Geometry check sheet. Reference: drawing and pictorial views, mm from the part's lowest x, y, z. Coordinates: 2 decimals unless noted, no trailing zeros. Order: outer loops, then holes, each group sorted by start corner. A loop starts at its lowest first (then second) coordinate and runs counter-clockwise, first axis right, second up. Notation, with made-up numbers: (85, 42.25) -> (99, 42.25) arc R21 ccw to (99, 52.25) -> close; hole circle Ø8 at (34, 34.5). An arc over 180 degrees is marked (long way). Use CSV: the item, a comma, the result in double quotes. Start each with the question number.
1) Sectioned sample at A-A on z = 3.75. Record the boundary of the cut face in (x, y).
2) Scan lines: line 1 along X through (y, z) = (7.5, 3.95); line 2 along Y through (x, z) = (31, 3.8); line 3 along Z through (x, y) = (17, 15). Record each from-to range of solid material in increasing order.
3) Sectioned sample at B-B on x = 38. Record the boundary of the cut face in (y, z), then the cut area to 3 significant figures.
4) Sectioned sample at D-D on x = 25. Record the boundary of the cut face in (y, z).
5) Go/stop test with flat-tipped pins: pin 1 (2 mm diameter, centred on x = 12.5, z = 3, fed in from -Y); pin 2 (6 mm diameter, centred on x = 15.5, y = 16, fed in from +Z); pin 3 (2 mm diameter, centred on x = 20, z = 1.5, fed in from +Y); pin 4 (1 mm diameter, centred on y = 29.5, z = 1.5, fed in from -X). Record where each tip stops, or that it passes through.
6) Release check for a two-part mould opening along X. For the marked faces 1, 2, 3 and 4 record: released by +X, released by -X, zero draft, split by the parting line, or undercut.
7) Sectioned sample at C-C on y = 11.5. Record the boundary of the cut face in (x, z), then the cut area to 3 significant figures.
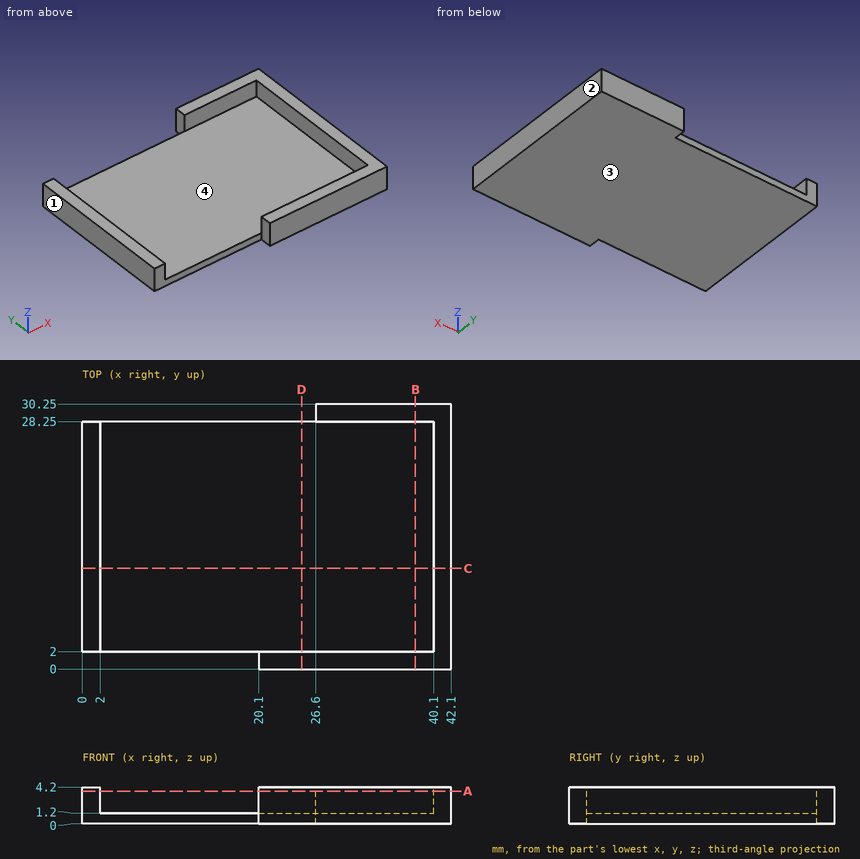
Answers follow:
1,outline,"(0, 2) -> (2, 2) -> (2, 28.25) -> (0, 28.25) -> close; (20.1, 0) -> (42.1, 0) -> (42.1, 30.25) -> (26.6, 30.25) -> (26.6, 28.25) -> (40.1, 28.25) -> (40.1, 2) -> (20.1, 2) -> close"
2,line 1,"x = 0 to 2, 40.1 to 42.1"
2,line 2,"y = 0 to 2, 28.25 to 30.25"
2,line 3,"z = 0 to 1.2"
3,outline,"(0, 0) -> (30.25, 0) -> (30.25, 4.2) -> (28.25, 4.2) -> (28.25, 1.2) -> (2, 1.2) -> (2, 4.2) -> (0, 4.2) -> close"
3,area,"48.3 mm²"
4,outline,"(0, 0) -> (28.25, 0) -> (28.25, 1.2) -> (2, 1.2) -> (2, 4.2) -> (0, 4.2) -> close"
5,pin 1,"passes through"
5,pin 2,"stops at z = 1.2"
5,pin 3,"stops at y = 28.25"
5,pin 4,"stops at x = 26.6"
6,face 1,"released by -X"
6,face 2,"released by +X"
6,face 3,"zero draft"
6,face 4,"undercut"
7,outline,"(0, 0) -> (42.1, 0) -> (42.1, 4.2) -> (40.1, 4.2) -> (40.1, 1.2) -> (2, 1.2) -> (2, 4.2) -> (0, 4.2) -> close"
7,area,"62.5 mm²"
